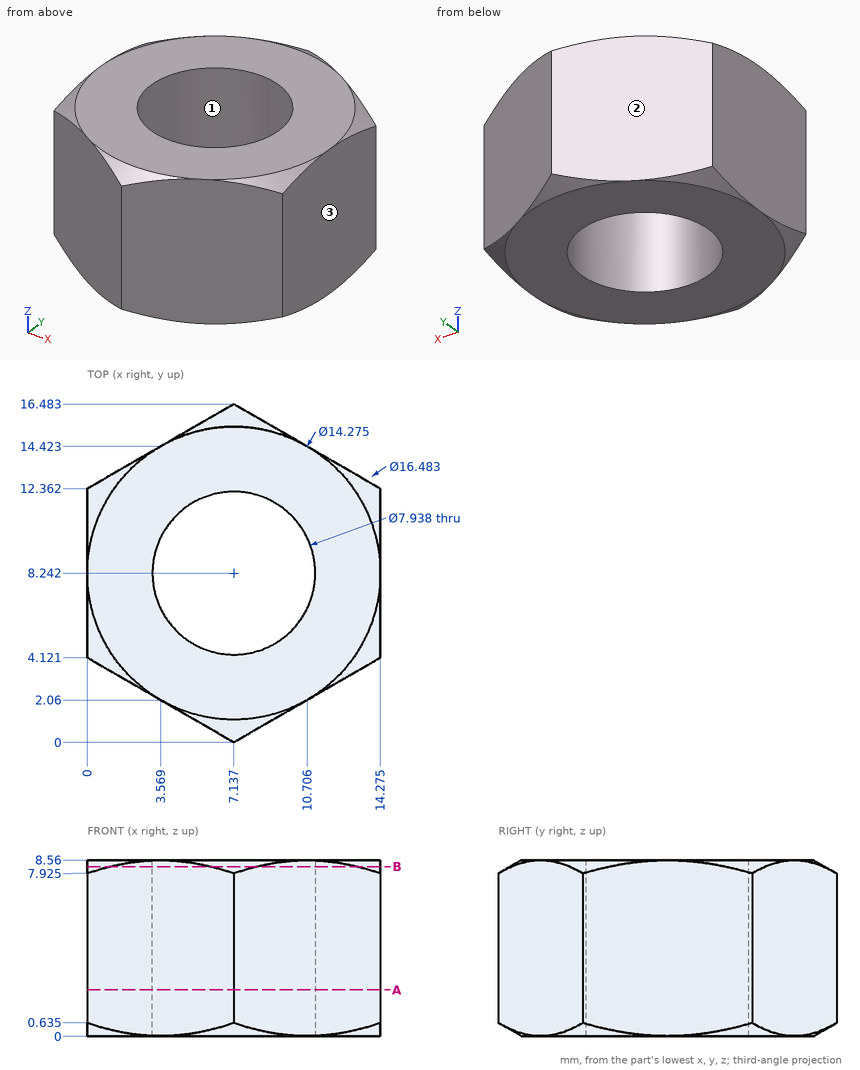
Geometry check sheet. Reference: drawing and pictorial views, mm from the part's lowest x, y, z. Give positions to 0.01 mm unless a question says otherwise; leave off trailing zeros. Order: outer loops, then holes, each group sorted by start corner. A loop starts at its lowest first (then second) coordinate and runs counter-clockwise, first axis right, second up. Notation, with made-up numbers: M -6,77 L 0,77 A21 cw 0,91 Z; hole C -10.5,26.5 d8. An arc over 180 degrees is marked long. Return JSON: item names as keys, results as strings. Group by question number.
1) Section check A-A on z = 2.25. Record the cut outline in (x, y) (1 decimal), and give its area (3 significant figures).
2) Section check B-B on z = 8.25. Record the cut outline in (x, y) (1 decimal).
3) Mould release check, pull along Y, two halves, no side actions. Record for the marked faces 1, 2 and 3: pulls with the +Y half, pulls with the -Y half, needs draft (parallel to the pull), parting line crosses it, or undercut.
4) Scan lines: line 1 (X direction, y = 10.75, z = 1) (1 decimal); line 2 (X direction, y = 11, z = 7.5) (1 decimal); line 3 (Y direction, x = 4.75, z = 3.5) (1 decimal). Record each from-to range of solid material in increasing order.
5) Go/stop test with flat-tipped pins: pin 1 Ø5 at (x, z) = (5, 5) entering from +Y; pin 2 Ø6.5 at (x, y) = (7.14, 8.24) entering from -Z; pin 3 Ø4 at (x, z) = (2.5, 4) entering from +Y; pin 4 Ø5 at (x, z) = (4.5, 7) entering from -Y. Record where each tip stops, or that it passes through.
Answer block:
{
 "1": {"outline": "M 0,4.1 L 7.1,0 L 14.3,4.1 L 14.3,12.4 L 7.1,16.5 L 0,12.4 Z; hole C 7.1,8.2 d7.9", "area": "127 mm^2"},
 "2": {"outline": "M 0,5.4 A7.7 ccw 1.1,3.5 L 6,0.6 A7.7 ccw 8.3,0.6 L 13.2,3.5 A7.7 ccw 14.3,5.4 L 14.3,11.1 A7.7 ccw 13.2,13 L 8.3,15.8 A7.7 ccw 6,15.8 L 1.1,13 A7.7 ccw 0,11.1 Z; hole C 7.1,8.2 d7.9"},
 "3": {"face 1": "undercut", "face 2": "pulls with the +Y half", "face 3": "needs draft"},
 "4": {"line 1": "x = 0 to 4.1, 10.2 to 14.3", "line 2": "x = 0 to 4.3, 10 to 14.3", "line 3": "y = 1.4 to 5.1, 11.4 to 15.1"},
 "5": {"pin 1": "stops at y = 16.48", "pin 2": "passes through", "pin 3": "stops at y = 14.96", "pin 4": "stops at y = 0.08"}
}
